CAD build for the part. Positions are in the model's coordinates, mm. Give positions to 0.01 mm unless a question says otherwise; leave off trailing zeros. Loops run counter-clockwise (first coordinate to the right, second up) from the corner with the lowest first, then second, coordinate; pieces in that order, holes last. Notation, with made-up numbers: M 25.25,62.25 L 59.25,62.25 A12 cw 59.25,85.25 Z; hole C 22,78 d9. An arc over 180 degrees is marked long. Answer as CSV lines item,"result".
```python
from build123d import *

# Parameters (mm, degrees)
ESQUISSE1_W             = 300
ESQUISSE1_H             = 300
BOSS_EXTRU_1_DEPTH      = 8
ESQUISSE3_W             = 8
ESQUISSE3_H             = 15
ENL_V_MAT_EXTRU_4_DEPTH = 213.282830205


with BuildPart() as part:
    # Esquisse1 → Boss.-Extru.1 (new body)
    with BuildSketch(Plane.XY):
        Rectangle(ESQUISSE1_W, ESQUISSE1_H)
    extrude(amount=BOSS_EXTRU_1_DEPTH)

    # Esquisse3 → Enlèv. mat.-Extru.4 (cut, through all)
    with BuildSketch(Plane.XY):
        with Locations((-146, -22.5)):
            Rectangle(ESQUISSE3_W, ESQUISSE3_H)
        with Locations((-146, -52.5)):
            Rectangle(ESQUISSE3_W, ESQUISSE3_H)
        with Locations((-146, -82.5)):
            Rectangle(ESQUISSE3_W, ESQUISSE3_H)
        with Locations((-146, -112.5)):
            Rectangle(ESQUISSE3_W, ESQUISSE3_H)
        with Locations((-146, -142.5)):
            Rectangle(ESQUISSE3_W, ESQUISSE3_H)
        with Locations((-146, 52.5)):
            Rectangle(ESQUISSE3_W, ESQUISSE3_H)
        with Locations((-146, 142.5)):
            Rectangle(ESQUISSE3_W, ESQUISSE3_H)
        with Locations((-146, 112.5)):
            Rectangle(ESQUISSE3_W, ESQUISSE3_H)
        with Locations((-146, 82.5)):
            Rectangle(ESQUISSE3_W, ESQUISSE3_H)
        with Locations((-146, 22.5)):
            Rectangle(ESQUISSE3_W, ESQUISSE3_H)
    enl_v_mat_extru_4 = extrude(amount=ENL_V_MAT_EXTRU_4_DEPTH, mode=Mode.SUBTRACT)

    # Symétrie1: Enlèv. mat.-Extru.4 across plane
    add(enl_v_mat_extru_4.mirror(Plane(origin=(0, 0, 0), x_dir=(0, 0, 1), z_dir=(1, 0, 0))), mode=Mode.SUBTRACT)


solid = part.part
```
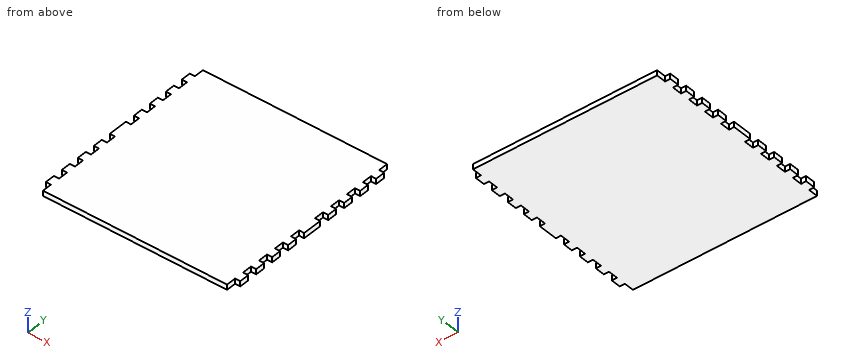
Q1. Pin check, flat tips, straight feed: P1, Ø4, axis at x = 145.5, z = 4.5, coming from the -Y side; P2, Ø2.5, axis at x = -147, z = 4, coming from the +Y side; P3, Ø2.5, axis at y = 55, z = 4, coming from the -X side; P4, Ø8, axis at x = -66.5, y = 28.5, coming from the -Z side. Stop position of each tip, or through.
Solution:
P1,"stops at y = -135"
P2,"stops at y = 135"
P3,"stops at x = -142"
P4,"stops at z = 0"
Q2. Cut at A-A (y = -115). Write the cut outline in (x, z).
Solution:
outline,"M -142,0 L 142,0 L 142,8 L -142,8 Z"
Q3. Wall check: line 1 (X direction, y = 29, z = 0.5). Give the ranges that are in metal, low to high. Write a range as [from, to].
Solution:
line 1,"x = [-142, 142]"
